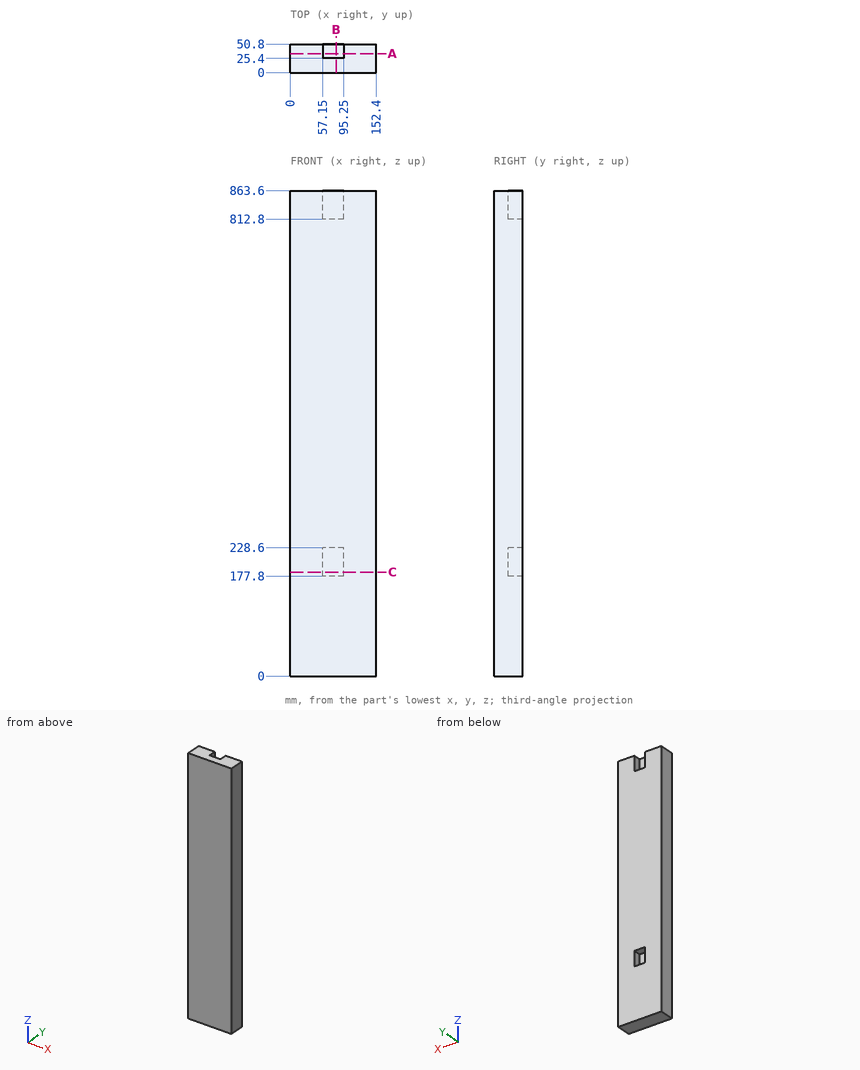
The figure shows three views and two pictorial views of one solid part (mm, origin at its lowest corner). Answer the questions. Coordinates: 2 decimals unless noted, no trailing zeros. Loops run counter-clockwise (first coordinate to the right, second up) from the corner with the lowest first, then second, coordinate; pieces in that order, holes last. Notation, with made-up numbers: M 74.25,10.25 L 91.25,10.25 A7 ccw 91.25,19.25 Z; hole C 13,28 d10. An arc over 180 degrees is marked long. Answer as CSV lines item,"result". Start each with the question number.
(1) Given pin 1 (2 mm diameter, centred on x = 118, y = 20.5, fed in from -Z); pin 2 (7.5 mm diameter, centred on x = 69, y = 41.5, fed in from +Z); pin 3 (19 mm diameter, centred on x = 73, z = 841.5, fed in from +Y), each flat-ended and moving along its own axis, determine where each tip first touches the part or whether it passes through.
(2) The part is cut by section B-B (x = 81.5). Give the vertices of the cut face in (y, z), and give its area (3 significant figures).
(3) The part is cut by section C-C (z = 185). Give the vertices of the cut face in (x, y).
(4) Find the intervals of material crossed by L1, parallel to X at y = 35, z = 198.5; L2, parallel to Z at x = 60.5, y = 28, in increasing order. Write a range as [from, to].
(5) The part is cut by section A-A (y = 33.5). Give the vertices of the cut face in (x, z), and give its area (3 significant figures).
Determined:
1,pin 1,"z = 0"
1,pin 2,"z = 812.8"
1,pin 3,"y = 25.4"
2,outline,"M 0,0 L 50.8,0 L 50.8,177.8 L 25.4,177.8 L 25.4,228.6 L 50.8,228.6 L 50.8,812.8 L 25.4,812.8 L 25.4,863.6 L 0,863.6 Z"
2,area,"41,300 mm2"
3,outline,"M 0,0 L 152.4,0 L 152.4,50.8 L 95.25,50.8 L 95.25,25.4 L 57.15,25.4 L 57.15,50.8 L 0,50.8 Z"
4,L1,"[0, 57.15], [95.25, 152.4]"
4,L2,"[0, 177.8], [228.6, 812.8]"
5,outline,"M 0,0 L 152.4,0 L 152.4,863.6 L 95.25,863.6 L 95.25,812.8 L 57.15,812.8 L 57.15,863.6 L 0,863.6 Z; hole M 57.15,177.8 L 95.25,177.8 L 95.25,228.6 L 57.15,228.6 Z"
5,area,"128,000 mm2"
